Build history of the part. All positions in model axes, mm. Round coordinates to 2 decimals unless told otherwise and drop trailing zeros. Loops run counter-clockwise (first coordinate to the right, second up) from the corner with the lowest first, then second, coordinate; pieces in that order, holes last.
from build123d import *

# Parameters (mm, degrees)
F0_W      = 40
F0_H      = 40
F1_DEPTH  = 600
F2_R      = 3
F3_DEPTH  = 12
F4_R      = 3
F5_DEPTH  = 12
F7_DEPTH  = 600
F8_R      = 3
F9_DEPTH  = 12
F10_DEPTH = 12
F11_R     = 3
F12_DEPTH = 12


with BuildPart() as f1:
    # F0 (on Top) → F1 (new body)
    with BuildSketch(Plane.XY):
        with Locations((-32.4728810042, 32.3857110739)):
            Rectangle(F0_W, F0_H)
    extrude(amount=F1_DEPTH)

    # F2 (on face) → F3 (cut)
    with BuildSketch(Plane.YZ.offset(-12.4728810042)):
        with Locations((27.3857110739, 570)):
            Circle(F2_R)
    extrude(amount=-F3_DEPTH, mode=Mode.SUBTRACT)

    # F4 (on face) → F5 (cut)
    with BuildSketch(Plane(origin=(0, 52.3857110739, 0), x_dir=(-1, 0, 0), z_dir=(0, 1, 0))):
        with Locations((37.4728810042, 570)):
            Circle(F4_R)
    extrude(amount=-F5_DEPTH, mode=Mode.SUBTRACT)

    # F6 (on face) → F7 (cut)
    with BuildSketch(Plane.XY.offset(600)):
        with BuildLine():
            ThreePointArc((-47.5474812124, 12.3857110739), (-47.0872668168, 13.3390112528), (-46.9291592401, 14.3857110739))
            ThreePointArc((-46.9291592401, 14.3857110739), (-48.8190187951, 17.5198303656), (-52.4728810042, 17.3111108656))
            Line((-52.4728810042, 17.3111108656), (-52.4728810042, 12.3857110739))
            Line((-52.4728810042, 12.3857110739), (-47.5474812124, 12.3857110739))
        make_face()
    extrude(amount=-F7_DEPTH, mode=Mode.SUBTRACT)

    # F8 (on face) → F9 (cut)
    with BuildSketch(Plane.XY.offset(600)):
        with Locations((-32.4728810042, 32.3857110739)):
            Circle(F8_R)
    extrude(amount=-F9_DEPTH, mode=Mode.SUBTRACT)

    # F4 (on face) → F10 (cut)
    with BuildSketch(Plane(origin=(0, 52.3857110739, 0), x_dir=(-1, 0, 0), z_dir=(0, 1, 0))):
        with Locations((32.4728810042, 450)):
            Circle(F4_R)
    extrude(amount=-F10_DEPTH, mode=Mode.SUBTRACT)

    # F11 (on face) → F12 (cut)
    with BuildSketch(Plane(origin=(0, 52.3857110739, 0), x_dir=(-1, 0, 0), z_dir=(0, 1, 0))):
        with Locations((32.4728810042, 150)):
            Circle(F11_R)
    extrude(amount=-F12_DEPTH, mode=Mode.SUBTRACT)


solid = f1.part
(1) Pin check, flat tips, straight feed: P1, Ø3.5, axis at x = -37.47, z = 570, coming from the +Y side; P2, Ø5.5, axis at y = 27.39, z = 570, coming from the +X side. Stop position of each tip, or through.
Responses:
P1: stops at y = 40.39
P2: stops at x = -24.47
(2) Slice it at A-A on z = 39.5. List the corners of the cut face in (x, y).
Responses:
outline: (-52.47, 17.31) arc R3.54 cw to (-47.55, 12.39) - (-12.47, 12.39) - (-12.47, 52.39) - (-52.47, 52.39) - close
(3) Probe line 1 (X direction, y = 45, z = 150); line 2 (Z direction, x = -31.5, y = 47); line 3 (Z direction, x = -40, y = 47). List the from-to ranges inside material, lowest first.
Responses:
line 1: x = -52.47 to -35.47, -29.47 to -12.47
line 2: z = 0 to 147.16, 152.84 to 447.16, 452.84 to 600
line 3: z = 0 to 568.38, 571.62 to 600
